Here's how the part is built. I have some questions about the finished solid (model axes, mm). A direction names the side the tool comes from. Coordinates: 2 decimals unless noted, no trailing zeros. Write each loop counter-clockwise with the first axis right and the second up, starting at its lowest first coordinate (ties: lowest second). Pieces come first, ordered by that corner, then holes.
(1) Thinking about a two-plate mould opening in Z: for faces 3 (the flat face through (11, -4, 10)), 4 (the cylindrical face through (-0.7, -2.23, 7.12)), 5 (the flat face through (0, -3, 11)), which applies, released by +Z, released by -Z, zero draft, split by the parting line, or undercut?
(2) Imagine slicing it at C-C, the plane y = 8. List the corners of the cut face in (x, z) for me.
(3) Which directions (+Z, -Z, +X, -X, +Y, -Y) give clear straight access to the entire face, cutting with the end or side of a thin tool? Please do faces 1 (the cylindrical face through (11.59, -4.81, 10.49)), 2 (the cylindrical face through (-2.504, -11.275, 4.93)).
(4) Imagine slicing it at A-A, the plane x = 0. List the corners of the cut face in (y, z) for me.
(5) For pin 1 Ø2 at (x, z) = (4.5, 7.5) entering from +Y; pin 2 Ø6 at (y, z) = (-8.5, 7) entering from +X; pin 3 Ø6 at (y, z) = (6.5, 5) entering from -X, each with a flat end and sliding along its axis, tell me the tip position at first contact or that it passes through.
(6) Please list where these lines run through material, in increasing order: probe 1 along X at (y, z) = (-3, 1); probe 2 along Y at (x, z) = (-2.5, 7.5); probe 3 along X at (y, z) = (3.5, 7.25).
(7) Imagine slicing it at B-B, the plane x = -4.5. List the corners of the cut face in (y, z) for me, plus the area to 3 significant figures.
```python
from build123d import *

# Parameters (mm, degrees)
F0_R     = 11.55
F1_DEPTH = 10
F2_R     = 12.55
F2_R_2   = 11.55
F3_DEPTH = 1
F7_R     = 3.25
F8_DEPTH = 27.57


with BuildPart() as f1:
    # F0 (on Top) → F1 (new body)
    with BuildSketch(Plane.XY):
        Circle(F0_R)
    extrude(amount=F1_DEPTH)

    # F2 (on face) → F3 (join)
    with BuildSketch(Plane.XY.offset(10)):
        Circle(F2_R)
        Circle(F2_R_2, mode=Mode.SUBTRACT)
        Circle(F2_R_2)
    extrude(amount=F3_DEPTH)

    # F7 (on face) → F8 (cut)
    with BuildSketch(Plane(origin=(0, 8.195943, 14.779569), x_dir=(1, 0, 0), z_dir=(0, 0.484968, 0.874532))):
        with Locations((0, -2.230057)):
            Circle(F7_R)
    extrude(amount=-F8_DEPTH, mode=Mode.SUBTRACT)


solid = f1.part
```
Recorded:
1. face 3: released by -Z
1. face 4: undercut
1. face 5: released by +Z
2. outline: (-9.67, 10) - (-8.33, 10) - (-8.33, 0) - (8.33, 0) - (8.33, 10) - (9.67, 10) - (9.67, 11) - (-9.67, 11) - close
3. face 1: +Z, -Z
3. face 2: -Z
4. outline: (-12.55, 10) - (-11.55, 10) - (-11.55, 0) - (-6.27, 0) - (-0.17, 11) - (-12.55, 11) - close; (1.17, 0) - (11.55, 0) - (11.55, 10) - (12.55, 10) - (12.55, 11) - (7.27, 11) - close
5. pin 1: stops at y = 11.01
5. pin 2: stops at x = 10.16
5. pin 3: stops at x = -11.01
6. probe 1: x = -11.15 to -3.13, 3.13 to 11.15
6. probe 2: y = -11.28 to -0.77, 3.98 to 11.28
6. probe 3: x = -11.01 to -2.72, 2.72 to 11.01
7. outline: (-11.72, 10) - (-10.64, 10) - (-10.64, 0) - (10.64, 0) - (10.64, 10) - (11.72, 10) - (11.72, 11) - (-11.72, 11) - close
7. area: 236 mm2
